from build123d import *

# Parameters (mm, degrees)
SKETCH_W    = 31.4
SKETCH_H    = 26.7
PAD_DEPTH   = 25
THICKNESS_T = 1.2
SKETCH001_R = 12.75
HOLE_DEPTH  = 25


with BuildPart() as part:
    # Sketch → Pad (new body)
    with BuildSketch(Plane.XY):
        Rectangle(SKETCH_W, SKETCH_H)
    extrude(amount=PAD_DEPTH)

    # Thickness
    thickness_openings = [part.faces().sort_by_distance(p)[0] for p in [
        (0, 0, 25),
    ]]
    offset(amount=THICKNESS_T, openings=thickness_openings)

    # Sketch001 (on Face5 of Thickness) → Hole (cut)
    with BuildSketch(Plane.XY):
        Circle(SKETCH001_R)
    extrude(amount=-HOLE_DEPTH, mode=Mode.SUBTRACT)


solid = part.part
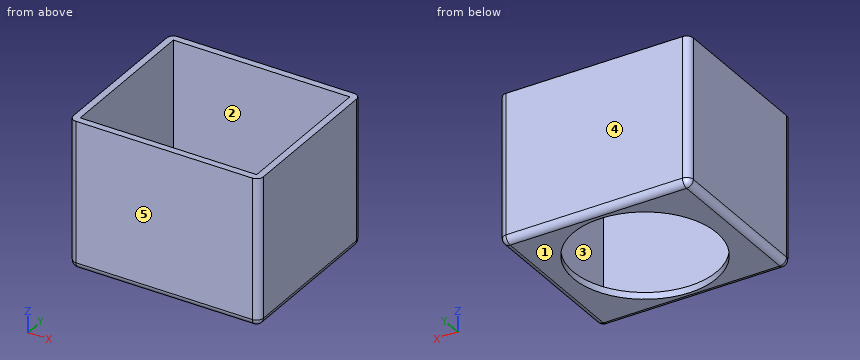
Geometry: final body of the model. Coordinates: model frame, mm. Face numbers are marked on the shaded views. A direction names the side the tool comes from. Give positions to 0.01 mm unless a question says otherwise; leave off trailing zeros. Write each loop counter-clockwise with the first axis right and the second up, starting at its lowest first coordinate (ties: lowest second). Pieces come first, ordered by that corner, then holes. Notation, with made-up numbers: M 34,48.25 L 51,48.25 A20 cw 51,54.25 Z; hole C -40,-30.75 d3. An arc over 180 degrees is marked long. Answer in a Markdown table with one row per item. Add a question column.
(1) Section C-C on z = 12.75. Return loops of the section in (x, y), and give its area (3 significant figures).
(2) Mould query, pull axis Y, two halves, no side actions, for the marked faces 3, 4 and 5. Classes: +Y half, -Y half, draft (parallel to the pull), parting line (faces both ways), or undercut.
(3) Ray query, line 1 (Y direction, x = 4, z = 4.5); line 2 (X direction, y = 2.75, z = 12.75); line 3 (Z direction, x = -14.5, y = -11.5). Return the intervals inside material, ascending.
(4) Reachability of the marked faces 1 and 2 from +Z, -Z, +X, -X, +Y, -Y: full face, straight path, thin tool, end or side. Return the list, or none.
(5) Section A-A on y = 0. Return loops of the section in (x, z), and give its area (3 significant figures).
(6) Section B-B on x = 0. Return loops of the section in (y, z), and give its area (3 significant figures).
(7) First-contact query: pin 1 (5 mm diameter, centred on x = -8, y = -6.5, fed in from +Z). Flat tip, straight axial feed; report the tip coordinate or a pass-through.
Result set:
| question | item | result |
|---|---|---|
| 1 | outline | M -16.9,-13.35 A1.2 ccw -15.7,-14.55 L 15.7,-14.55 A1.2 ccw 16.9,-13.35 L 16.9,13.35 A1.2 ccw 15.7,14.55 L -15.7,14.55 A1.2 ccw -16.9,13.35 Z; hole M -15.7,-13.35 L 15.7,-13.35 L 15.7,13.35 L -15.7,13.35 Z |
| 1 | area | 144 mm^2 |
| 2 | face 3 | undercut |
| 2 | face 4 | +Y half |
| 2 | face 5 | -Y half |
| 3 | line 1 | y = -14.55 to -13.35, 13.35 to 14.55 |
| 3 | line 2 | x = -16.9 to -15.7, 15.7 to 16.9 |
| 3 | line 3 | z = -1.2 to 0 |
| 4 | face 1 | -Z, +X, -X, +Y, -Y |
| 4 | face 2 | +Z |
| 5 | outline | M -16.9,0 A1.2 ccw -15.7,-1.2 L -12.75,-1.2 L -12.75,0 L -15.7,0 L -15.7,25 L -16.9,25 Z; M 12.75,-1.2 L 15.7,-1.2 A1.2 ccw 16.9,0 L 16.9,25 L 15.7,25 L 15.7,0 L 12.75,0 Z |
| 5 | area | 69.3 mm^2 |
| 6 | outline | M -14.55,0 A1.2 ccw -13.35,-1.2 L -12.75,-1.2 L -12.75,0 L -13.35,0 L -13.35,25 L -14.55,25 Z; M 12.75,-1.2 L 13.35,-1.2 A1.2 ccw 14.55,0 L 14.55,25 L 13.35,25 L 13.35,0 L 12.75,0 Z |
| 6 | area | 63.7 mm^2 |
| 7 | pin 1 | stops at z = 0 |
